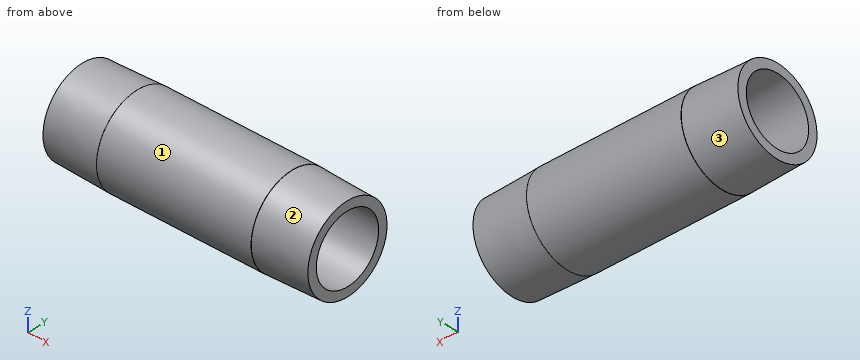
Autodesk Inventor part; units mm, degrees
ref_plane "YZ Plane" through (0, 0, 0) normal (1, 0, 0) x (0, 1, 0)
ref_plane "XZ Plane" through (0, 0, 0) normal (0, 1, 0) x (-1, 0, 0)
ref_plane "XY Plane" through (0, 0, 0) normal (0, 0, 1) x (1, 0, 0)
sketch "Sketch1" plane through (0, 0, 0) normal (0, 1, 0) x (-1, 0, 0)
  line L0 (-63.5, 0) -> (0, 0)
  line L1 (0, 0) -> (0, 8.05) construction
  line L2 (0, 8.05) -> (0, 10.2212)
  line L3 (0, 10.2212) -> (-13.2, 10.6337)
  line L4 (-13.2, 10.6337) -> (-13.2281, 10.65)
  line L5 (-13.2281, 10.65) -> (-50.2719, 10.65)
  line L6 (0, 8.05) -> (-63.5, 8.05)
  line L7 (-31.75, 0) -> (-31.75, 10.65) construction
  line L8 (-63.5, 0) -> (-63.5, 8.05) construction
  line L9 (-63.5, 8.05) -> (-63.5, 10.2212)
  line L10 (-63.5, 10.2212) -> (-50.3, 10.6337)
  line L11 (-50.3, 10.6337) -> (-50.2719, 10.65)
  line L12 (-8.2, 10.4775) -> (-8.2, 0) construction
  line L13 (-13.2, 10.6337) -> (-13.2, 0) construction
  line L14 (-50.3, 10.6337) -> (-50.3, 0) construction
  dimension "d0" = 8.2
  dimension "d1" = 13.2
  dimension "d2" = 1.79
  dimension "d3" = 20.955
  dimension "d4" = 21.3
  dimension "d5" = 2.6
  dimension "d6" = 63.5
  dimension "d7" = 30
revolve "Revolution1" add sketch "Sketch1" angle 360 about axis through (63.5, 0, 0) along (-1, 0, 0)
thread "Thread1"
thread "Thread2"
equation "\"d0\" = a"
equation "\"d1\" = LT"
equation "\"d3\" = MjD"
equation "\"d4\" = OD"
equation "\"d5\" = T"
equation "\"d6\" = L"
equation "\"OD\" = 21.3"
equation "\"T\" = 2.6"
equation "\"L\" = PL"
equation "\"LT\" = 13.2"
equation "\"ID\" = 16.1"
equation "\"PL\" = 63.5"
equation "\"MjD\" = 20.955"
equation "\"a\" = 8.2"
equation "\"Size_Designation\" = 1.2345"
equation "\"PLmin\" = 2 * LT + T"
properties material "Stainless Steel"
Geometry check sheet. Reference: the model listing, model coordinates, mm. Face numbers are marked on the shaded views. A direction names the side the tool comes from. Give positions to 0.01 mm unless a question says otherwise; leave off trailing zeros. Write each loop counter-clockwise with the first axis right and the second up, starting at its lowest first coordinate (ties: lowest second). Pieces come first, ordered by that corner, then holes. Notation, with made-up numbers: (61.5, 48.5) -> (84.5, 48.5) arc R17 cw to (84.5, 74.5) -> close; hole circle Ø9 at (87.5, 2). An arc over 180 degrees is marked (long way). Use one line per item in the form item = value.
Item 1: Sectioned sample at D-D on x = 51.5. Enter the section's corners in (y, z), plus the area to 3 significant figures.
Results list:
outline = circle Ø21.19 at (0, 0); hole circle Ø16.1 at (0, 0)
area = 149 mm2
Item 2: Depth check by flat-ended pin: pin 1 Ø5 at (y, z) = (4, 2) entering from +X; pin 2 Ø1.5 at (x, z) = (27, 5.5) entering from -Y; pin 3 Ø6 at (x, y) = (52.5, -5) entering from +Z; pin 4 Ø4 at (x, y) = (28.5, -8.5) entering from -Z. Enter the tip coordinate at first touch or a pass-through.
Results list:
pin_1 = through
pin_2 = -9.53
pin_3 = 10.38
pin_4 = -8.44
Item 3: Sectioned sample at C-C on x = 40. Enter the section's corners in (y, z), plus the area to 3 significant figures.
Results list:
outline = circle Ø21.3 at (0, 0); hole circle Ø16.1 at (0, 0)
area = 153 mm2
Item 4: Scan lines: line 1 (Y direction, x = 33.5, z = 0); line 2 (Z direction, x = 44, y = -2.75); line 3 (Y direction, x = 8.5, z = -2). Record each from-to range of solid material in increasing order.
Results list:
line_1 = -10.65 to -8.05, 8.05 to 10.65
line_2 = -10.29 to -7.57, 7.57 to 10.29
line_3 = -10.29 to -7.8, 7.8 to 10.29
Item 5: Access from +Z, -Z, +X, -X, +Y, -Y to the whole of each face (thin tool, end or side, straight path). Record for the marked faces 1, 2 and 3.
Results list:
face_1 = +X, -X
face_2 = +X
face_3 = -X
